```python
from build123d import *

# Parameters (mm, degrees)
SKETCH4_W                      = 72.837083297
SKETCH4_H                      = 43.95
BOSS_EXTRUDE1_DEPTH            = 8
BOSS_EXTRUDE2_DEPTH            = 14
SKETCH6_W                      = 30.477083297
SKETCH6_H                      = 2
SKETCH6_W_2                    = 33.837083297
BOSS_EXTRUDE3_DEPTH            = 6
CBORE_FOR_M4_SHCS1_D           = 4.5
CBORE_FOR_M4_SHCS1_CBORE_D     = 8
CBORE_FOR_M4_SHCS1_CBORE_DEPTH = 4
F_4_0MM_DOWEL_HOLE1_D          = 4
CUT_EXTRUDE1_DEPTH             = 3.4


with BuildPart() as part:
    # Sketch4 → Boss-Extrude1 (new body)
    with BuildSketch(Plane(origin=(0, 0, 0), x_dir=(1, 0, 0), z_dir=(0, 1, 0))):
        with Locations((-0.418541648, 0)):
            Rectangle(SKETCH4_W, SKETCH4_H)
    extrude(amount=BOSS_EXTRUDE1_DEPTH)

    # Sketch5 → Boss-Extrude2 (add)
    with BuildSketch(Plane(origin=(0, 8, 0), x_dir=(1, 0, 0), z_dir=(0, 1, 0))):
        Polygon((36, 13.975), (34, 13.975), (34, 19.975), (-36.837083297, 19.975), (-36.837083297, 21.975), (36, 21.975), align=None)
        Polygon((-36.837083297, -21.975), (36, -21.975), (36, -16.975), (34, -16.975), (34, -19.975), (-36.837083297, -19.975), align=None)
    extrude(amount=BOSS_EXTRUDE2_DEPTH)

    # Sketch6 → Boss-Extrude3 (add)
    with BuildSketch(Plane(origin=(0, 22, 0), x_dir=(1, 0, 0), z_dir=(0, 1, 0))):
        with Locations((-21.598541648, 20.975)):
            Rectangle(SKETCH6_W, SKETCH6_H)
        Polygon((36, 21.975), (27.64, 21.975), (27.64, 19.975), (34, 19.975), (34, 13.975), (36, 13.975), align=None)
        Polygon((36, -21.975), (27.43, -21.975), (27.43, -19.975), (34, -19.975), (34, -16.975), (36, -16.975), align=None)
        with Locations((-19.918541648, -20.975)):
            Rectangle(SKETCH6_W_2, SKETCH6_H)
    extrude(amount=BOSS_EXTRUDE3_DEPTH)

    # CBORE for M4 SHCS1 (through all)
    with Locations(Plane(origin=(0, 0, 0), x_dir=(-1, 0, 0), z_dir=(0, -1, 0))):
        with Locations((-2.85, 0), (-19, 16.42), (-19, -16.42)):
            CounterBoreHole(CBORE_FOR_M4_SHCS1_D / 2, CBORE_FOR_M4_SHCS1_CBORE_D / 2, CBORE_FOR_M4_SHCS1_CBORE_DEPTH)

    # Ø4.0mm Dowel Hole1 (through all)
    with Locations(Plane(origin=(0, 0, 0), x_dir=(-1, 0, 0), z_dir=(0, -1, 0))):
        with Locations((-12.84040165, 0.00815259), (27.15959835, 10.00815259), (27.15959835, -9.99184741)):
            Hole(F_4_0MM_DOWEL_HOLE1_D / 2)

    # Sketch12 → Cut-Extrude1 (cut)
    with BuildSketch(Plane(origin=(0, 8, 0), x_dir=(1, 0, 0), z_dir=(0, 1, 0))):
        Polygon((12.84040165, 4.049604475), (9.34040165, 2.028878533), (9.34040165, -2.012573352), (12.84040165, -4.033299294), (16.34040165, -2.012573352), (16.34040165, 2.028878533), align=None)
        Polygon((-27.15959835, 14.049604475), (-30.65959835, 12.028878533), (-30.65959835, 7.987426648), (-27.15959835, 5.966700706), (-23.65959835, 7.987426648), (-23.65959835, 12.028878533), align=None)
        Polygon((-27.15959835, -5.950395525), (-30.65959835, -7.971121467), (-30.65959835, -12.012573352), (-27.15959835, -14.033299294), (-23.65959835, -12.012573352), (-23.65959835, -7.971121467), align=None)
    extrude(amount=-CUT_EXTRUDE1_DEPTH, mode=Mode.SUBTRACT)


solid = part.part
```
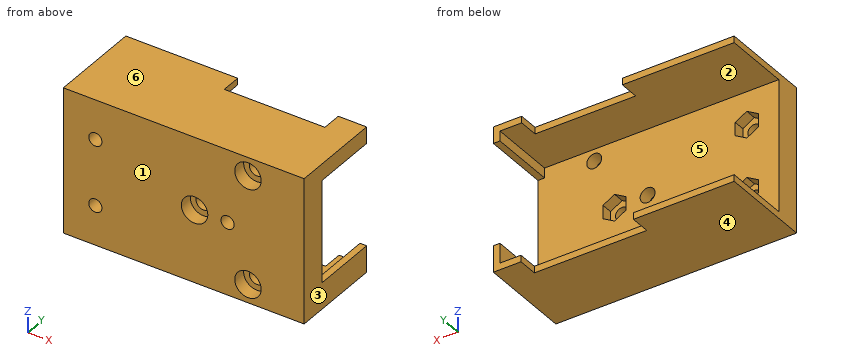
Check sheet for the modelled part. Datum: model origin and axes. Units: mm. Face numbers are marked on the shaded views. A direction names the side the tool comes from. Round coordinates to 2 decimals unless told otherwise and drop trailing zeros. Order: outer loops, then holes, each group sorted by start corner. A loop starts at its lowest first (then second) coordinate and runs counter-clockwise, first axis right, second up. Notation, with made-up numbers: (35.25, -16.5) -> (55.25, -16.5) arc R20 cw to (55.25, 1.5) -> close; hole circle Ø10 at (-7, -14.5). An arc over 180 degrees is marked (long way). Use CSV: the item, a comma, the result in double quotes.
(1) Cross-section at C-C (x = 19). Record the boundary of the cut face in (y, z) (3 decimals), and give its area (3 significant figures).
Worked out:
outline,"(0, -21.975) -> (22, -21.975) -> (22, -19.975) -> (8, -19.975) -> (8, -18.67) -> (4, -18.67) -> (4, -20.42) -> (0, -20.42) -> close; (0, -12.42) -> (4, -12.42) -> (4, -14.17) -> (8, -14.17) -> (8, 14.17) -> (4, 14.17) -> (4, 12.42) -> (0, 12.42) -> close; (0, 20.42) -> (4, 20.42) -> (4, 18.67) -> (8, 18.67) -> (8, 19.975) -> (22, 19.975) -> (22, 21.975) -> (0, 21.975) -> close"
area,"308 mm²"
(2) Tool access check on the marked faces 1 and 2. Record the directions out of +Z, -Z, +X, -X, +Y, -Y that give a thin tool (end or side, any length) a straight path to the whole face; none if there is none.
Worked out:
face 1,"+Z, -Z, +X, -X, -Y"
face 2,"-X, +Y"
(3) Cross-section at A-A (x = 2.85). Record the boundary of the cut face in (y, z) (3 decimals).
Worked out:
outline,"(0, -21.975) -> (22, -21.975) -> (22, -19.975) -> (8, -19.975) -> (8, -2.25) -> (4, -2.25) -> (4, -4) -> (0, -4) -> close; (0, 4) -> (4, 4) -> (4, 2.25) -> (8, 2.25) -> (8, 19.975) -> (22, 19.975) -> (22, 21.975) -> (0, 21.975) -> close"
(4) Draft check along Z on the marked faces 3, 4, 5 and 6. Enter one of: pulls with the +Z half, pulls with the -Z half, needs draft (parallel to the pull), parting line crosses it, or undercut.
Worked out:
face 3,"needs draft"
face 4,"pulls with the -Z half"
face 5,"undercut"
face 6,"pulls with the +Z half"
(5) Cross-section at D-D (y = 24.5). Record the boundary of the cut face in (x, z) (3 decimals), and give its area (3 significant figures).
Worked out:
outline,"(-36.837, -21.975) -> (-6.36, -21.975) -> (-6.36, -19.975) -> (-36.837, -19.975) -> close; (-36.837, 19.975) -> (-3, 19.975) -> (-3, 21.975) -> (-36.837, 21.975) -> close; (27.43, 19.975) -> (34, 19.975) -> (34, 16.975) -> (36, 16.975) -> (36, 21.975) -> (27.43, 21.975) -> close; (27.64, -21.975) -> (36, -21.975) -> (36, -13.975) -> (34, -13.975) -> (34, -19.975) -> (27.64, -19.975) -> close"
area,"180 mm²"
(6) Depth check by flat-ended pin: pin 1 (8 mm diameter, centred on y = 13.5, z = -12.5, fed in from +X); pin 2 (2 mm diameter, centred on x = 12, z = 2, fed in from +Y); pin 3 (2 mm diameter, centred on x = 20, z = -9, fed in from +Y); pin 4 (0.9 mm diameter, centred on y = 20.5, z = 18.5, fed in from -X). Enter the tip coordinate at first touch or a pass-through.
Worked out:
pin 1,"x = 36"
pin 2,"y = 4.6"
pin 3,"y = 8"
pin 4,"x = 34"
(7) Cross-section at B-B (y = 9.5). Record the boundary of the cut face in (x, z) (3 decimals).
Worked out:
outline,"(-36.837, -21.975) -> (36, -21.975) -> (36, -13.975) -> (34, -13.975) -> (34, -19.975) -> (-36.837, -19.975) -> close; (-36.837, 19.975) -> (34, 19.975) -> (34, 16.975) -> (36, 16.975) -> (36, 21.975) -> (-36.837, 21.975) -> close"
(8) Material ranges on line 1 along Z through (x, y) = (19, 6.05) (3 decimals); line 2 along Z through (x, y) = (19, 2.8) (3 decimals); line 3 along Z through (x, y) = (2.85, 1.1) (3 decimals), recorded low to high. Write a range as from..to.
Worked out:
line 1,"-21.975..-18.67, -14.17..14.17, 18.67..21.975"
line 2,"-21.975..-20.42, -12.42..12.42, 20.42..21.975"
line 3,"-21.975..-4, 4..21.975"
